from build123d import *

# Parameters (mm, degrees)
F0_R        = 1.5
F0_R_2      = 1.3
F1_DEPTH    = 39.5
F2_DEPTH    = 1
F3_START    = -0.5
F3_DEPTH    = 0.5
F4_R        = 1.3
F5_DEPTH    = 1
F6_START    = 0.5
F1_FACE_R   = 1.5
F1_FACE_R_2 = 1.3
F6_DEPTH    = 0.5
F7_SIZE     = 0.2
F8_SIZE     = 0.1


with BuildPart() as f1:
    # F0 (on Top) → F1 (new body)
    with BuildSketch(Plane.XY):
        Circle(F0_R)
        Circle(F0_R_2, mode=Mode.SUBTRACT)
        Circle(F0_R_2)
    extrude(amount=F1_DEPTH)

    # F0 (on Top) → F2 (join)
    with BuildSketch(Plane.XY):
        Circle(F0_R_2)
    extrude(amount=-F2_DEPTH)

    # F0 (on Top) → F3 (join)
    with BuildSketch(Plane.XY.offset(F3_START)):
        Circle(F0_R)
        Circle(F0_R_2, mode=Mode.SUBTRACT)
    extrude(amount=-F3_DEPTH)

    # F4 (on face) → F5 (join)
    with BuildSketch(Plane.XY.offset(39.5)):
        Circle(F4_R)
    extrude(amount=F5_DEPTH)

    # F1_face (on face) → F6 (join)
    with BuildSketch(Plane.XY.offset(39.5).offset(F6_START)):
        Circle(F1_FACE_R)
        Circle(F1_FACE_R_2, mode=Mode.SUBTRACT)
    extrude(amount=F6_DEPTH)

    # F7
    f7_edges = [f1.edges().sort_by_distance(p)[0] for p in [
        (-1.5, 0, -1),
        (-1.5, 0, 40.5),
    ]]
    chamfer(f7_edges, length=F7_SIZE)

    # F8
    f8_edges = [f1.edges().sort_by_distance(p)[0] for p in [
        (-1.5, 0, -0.5),
        (-1.5, 0, 0),
        (-1.5, 0, 39.5),
        (-1.5, 0, 40),
    ]]
    chamfer(f8_edges, length=F8_SIZE)


solid = f1.part
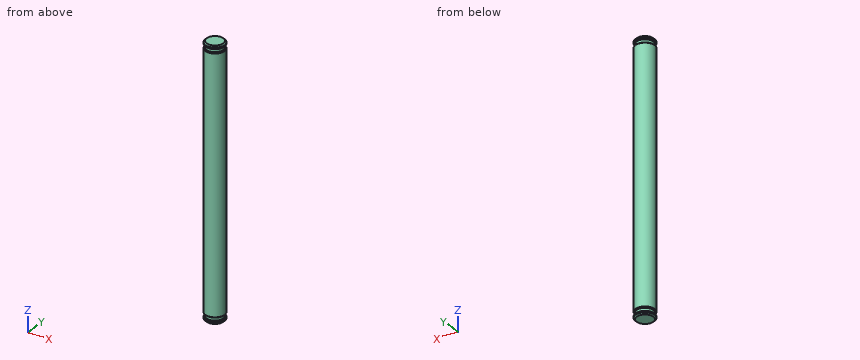
Design review of the part built by this model. Coordinates are the model's own, in mm. Round coordinates to 2 decimals unless told otherwise and drop trailing zeros. Loops run counter-clockwise (first coordinate to the right, second up) from the corner with the lowest first, then second, coordinate; pieces in that order, holes last. Notation, with made-up numbers: (-31.75, 52) -> (17.25, 52) arc R20 ccw to (17.25, 88) -> close; hole circle Ø9 at (-7, 85). An arc over 180 degrees is marked (long way). Use one line per item in the form item = value. Start each with the question number.
Q1. Wall thickness on line 1 along Z through (x, y) = (1.25, 0.45); line 2 along X through (y, z) = (-0.1, 20); line 3 along Y through (x, z) = (0.15, 1.5): over which ranges is each line inside the solid? List them lowest first. Write a range as [from, to].
Q2. We need section A-A on z = 26.5. Give the boundary of the cut face in (x, y).
Q3. For pin 1 Ø1.5 at (y, z) = (1, 17) entering from +X, flat-tipped, find the tip position at first contact; note if it passes through.
Calculated:
q1.line_1 = [-0.97, -0.5], [0, 39.5], [40, 40.47]
q1.line_2 = [-1.5, 1.5]
q1.line_3 = [-1.49, 1.49]
q2.outline = circle Ø3 at (0, 0)
q3.pin_1 = 1.48
